Geometry: see drawing. Coordinates: mm, zero at the bounding-box minimum. Round coordinates to 2 decimals unless told otherwise and drop trailing zeros. Loops run counter-clockwise (first coordinate to the right, second up) from the corner with the lowest first, then second, coordinate; pieces in that order, holes last. Notation, with made-up numbers: (86.5, 65.5) - (95.5, 65.5) arc R5 cw to (95.5, 73.5) - close; hole circle Ø4 at (52, 44.25). An arc over 180 degrees is marked (long way). Write item = value, one per line. Start each with the question number.
Item 1: Draft query along X for the marked faces 1, 2, 3 and 4. Return one class per face: pulls with the +X half, pulls with the -X half, needs draft (parallel to the pull), parting line crosses it, or undercut.
Item 2: First-contact query: pin 1 (0.8 mm diameter, centred on x = 23, z = 9.5, fed in from -Y); pin 2 (7 mm diameter, centred on x = 17.25, z = 9, fed in from +Y); pin 3 (0.8 mm diameter, centred on x = 4.5, z = 8, fed in from -Y). Flat tips, straight axial feed; report the tip coordinate or a pass-through.
Item 3: Section C-C (y = 45.5). Return loops of the section in (x, z), plus the area to 3 significant figures.
Item 4: Line query: line 1 (Z direction, x = 17, y = 46) (3 decimals); line 2 (Y direction, x = 7.75, z = 9); line 3 (Y direction, x = 4.75, z = 9). Output: solid intervals per line, ascending. Write a range as from..to.
Item 5: Section A-A (y = 53). Return loops of the section in (x, z).
Item 6: Section B-B (x = 30). Return loops of the section in (y, z).
Item 7: Section D-D (z = 10). Count the separate pieces of the cut face and the enclosed holes in it, plus the area to 3 significant figures.
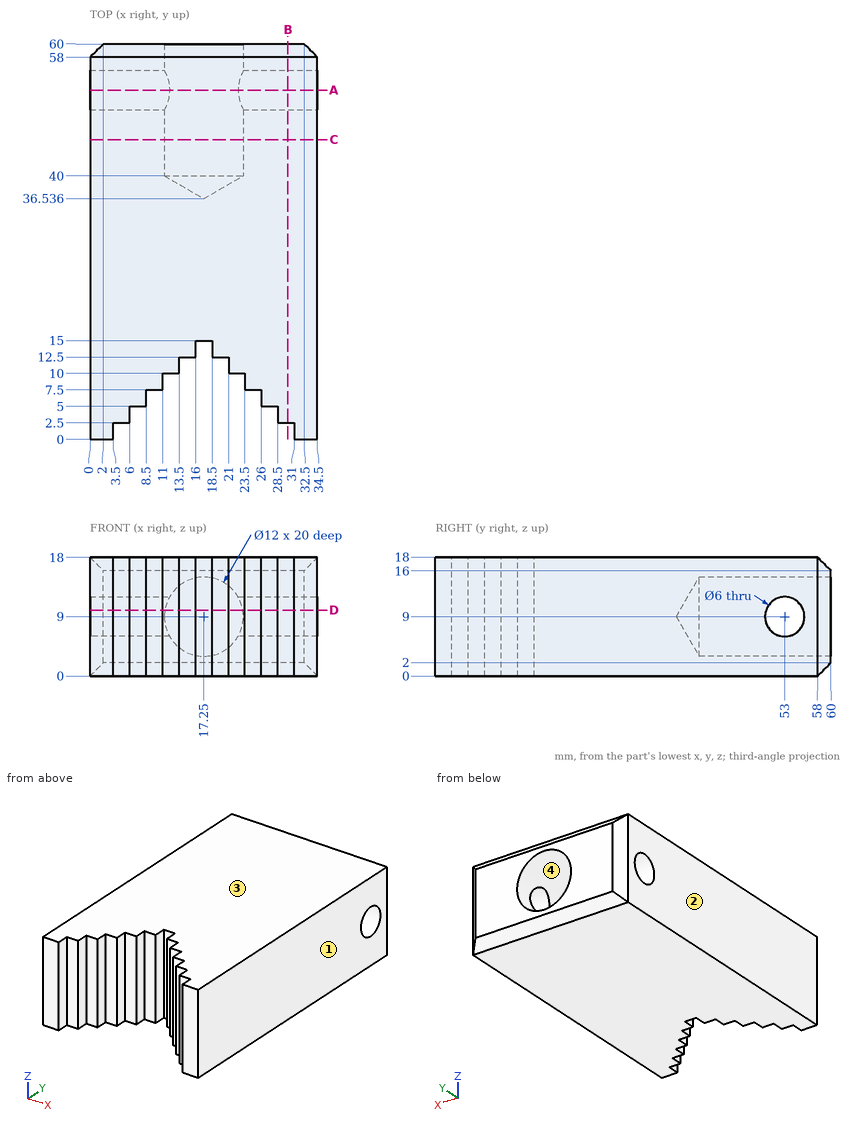
Taken from the geometry:
q1.face_1 = pulls with the +X half
q1.face_2 = pulls with the -X half
q1.face_3 = needs draft
q1.face_4 = undercut
q2.pin_1 = 10
q2.pin_2 = 38.56
q2.pin_3 = 2.5
q3.outline = (0, 0) - (34.5, 0) - (34.5, 18) - (0, 18) - close; hole circle Ø12 at (17.25, 9)
q3.area = 508 mm^2
q4.line_1 = 0..3.005, 14.995..18
q4.line_2 = 5..50, 56..60
q4.line_3 = 2.5..50, 56..60
q5.outline = (0, 0) - (34.5, 0) - (34.5, 6) - (22.45, 6) arc R6 cw to (12.05, 6) - (0, 6) - close; (0, 12) - (12.05, 12) arc R6 cw to (22.45, 12) - (34.5, 12) - (34.5, 18) - (0, 18) - close
q6.outline = (2.5, 0) - (58, 0) - (60, 2) - (60, 16) - (58, 18) - (2.5, 18) - close; hole circle Ø6 at (53, 9)
q7.separate_pieces = 3
q7.enclosed_holes = 0
q7.area = 1,460 mm^2
